The figure shows three views and two pictorial views of one solid part (mm, origin at its lowest corner). Answer the questions. A direction names the side the tool comes from. Round coordinates to 2 decimals unless told otherwise and drop trailing zeros. Write each loop counter-clockwise with the first axis right and the second up, starting at its lowest first coordinate (ties: lowest second). Pieces come first, ordered by that corner, then holes. Notation, with made-up numbers: M 86.5,-30.5 L 101.5,-30.5 A14 cw 101.5,-10.5 Z; hole C -22.5,74.25 d8. An arc over 180 degrees is marked long. Answer in a Markdown table with one row per item.
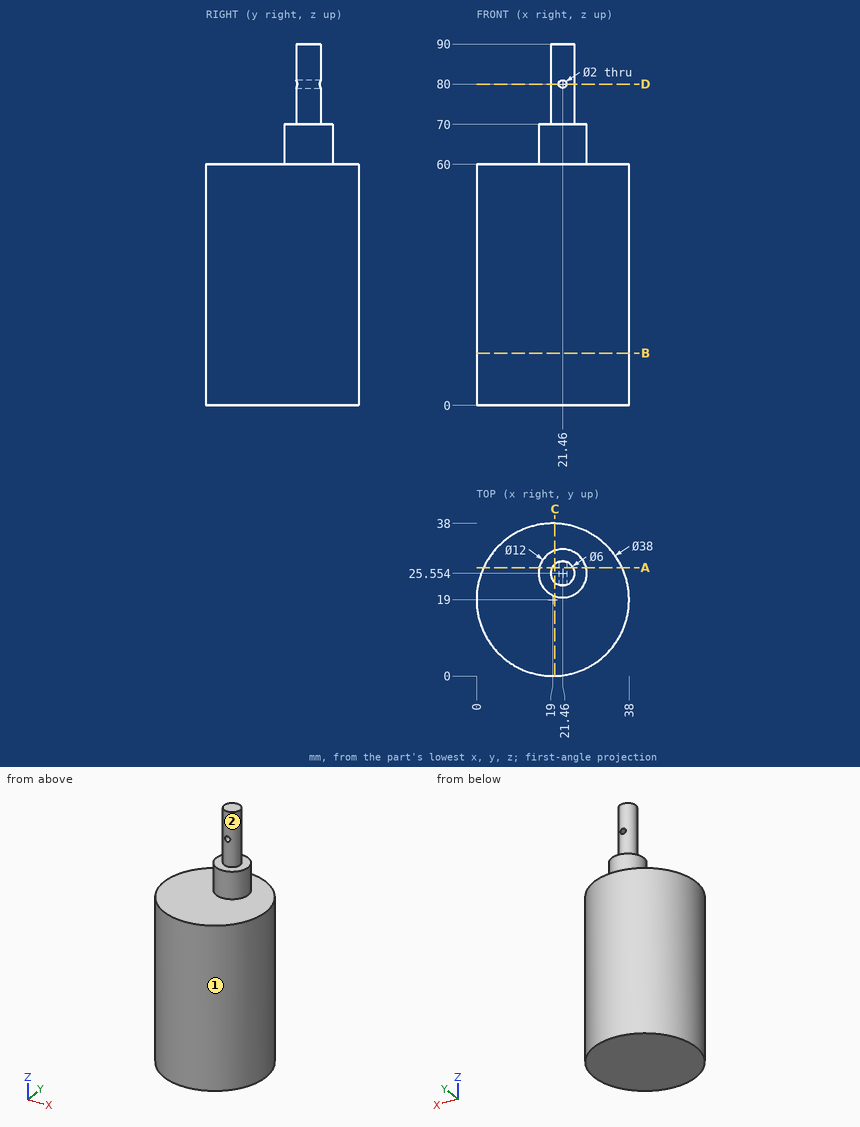
1. The part is cut by section A-A (y = 27). Determine the outline of the cut face in (x, z), plus the area to 3 significant figures.
Calculated:
| item | result |
|---|---|
| outline | M 1.77,0 L 36.23,0 L 36.23,60 L 27.28,60 L 27.28,70 L 24.09,70 L 24.09,90 L 18.83,90 L 18.83,70 L 15.64,70 L 15.64,60 L 1.77,60 Z; hole C 21.46,80 d2 |
| area | 2,290 mm² |
2. Consider line 1 along X through (y, z) = (25.75, 80); line 2 along Z through (x, y) = (22, 4.5); line 3 along Z through (x, y) = (18.5, 24). Determine where each line is inside the solid, lowest interval first. Write a range as from..to.
Calculated:
| item | result |
|---|---|
| line 1 | x = 18.47..20.46, 22.46..24.45 |
| line 2 | z = 0..60 |
| line 3 | z = 0..70 |
3. Given pin 1 (1 mm diameter, centred on y = 21, z = 69, fed in from +X); pin 2 (1 mm diameter, centred on y = 24, z = 73, fed in from -X); pin 3 (10 mm diameter, centred on y = 24.5, z = 71, fed in from +X), each flat-ended and moving along its own axis, determine where each tip first touches the part or whether it passes through.
Calculated:
| item | result |
|---|---|
| pin 1 | stops at x = 25.88 |
| pin 2 | stops at x = 18.65 |
| pin 3 | stops at x = 27.46 |
4. The part is cut by section C-C (x = 19.5). Determine the outline of the cut face in (y, z) (1 decimal), plus the area to 3 significant figures.
Calculated:
| item | result |
|---|---|
| outline | M 0,0 L 38,0 L 38,60 L 31.2,60 L 31.2,70 L 27.8,70 L 27.8,90 L 23.3,90 L 23.3,70 L 19.9,70 L 19.9,60 L 0,60 Z |
| area | 2,480 mm² |
5. The part is cut by section B-B (z = 13). Determine the outline of the cut face in (x, y), plus the area to 3 significant figures.
Calculated:
| item | result |
|---|---|
| outline | C 19,19 d38 |
| area | 1,130 mm² |
6. The part is cut by section D-D (z = 80). Determine the outline of the cut face in (x, y) (1 decimal).
Calculated:
| item | result |
|---|---|
| outline | M 20.5,22.7 L 20.5,28.4 A3 ccw Z; M 22.5,22.7 A3 ccw 22.5,28.4 Z |
7. A tool of negligible diameter and unlimited length cuts with its end or side. For the marked faces 1 and 2, from which of +Z, -Z, +X, -X, +Y, -Y can it reach the whole face along a straight path? Write none if from no direction.
Calculated:
| item | result |
|---|---|
| face 1 | +Z, -Z |
| face 2 | +Z |
